Could you check a few things on this drawing? It's one solid part, dimensions in mm from its lowest x, y, z. Give positions to 0.01 mm unless a question says otherwise; leave off trailing zeros. Loops run counter-clockwise (first coordinate to the right, second up) from the corner with the lowest first, then second, coordinate; pieces in that order, holes last. Notation, with made-up numbers: M -22.5,-2 L -17.5,-2 A10 cw -17.5,4 Z; hole C 25,30.5 d2. An arc over 180 degrees is marked long. Return JSON: item names as keys, results as strings. Group by question number.
1. Please list where this line runs through material, in increasing order: line 1 (Y direction, x = 31, z = 0.6).
2. For pin 1 (10 mm diameter, centred on x = 127.5, y = 36, fed in from -Z); pin 2 (2 mm diameter, centred on x = 68, y = 32.5, fed in from +Z), each with a flat end and sliding along its axis, tell me the tip position at first contact or that it passes through.
3. If we section it at A-A (y = 34.5): State how many separate pieces and enclosed holes the cut face has.
4. If we section it at B-B (x = 131): Write out the boundary of the cut face in (y, z).
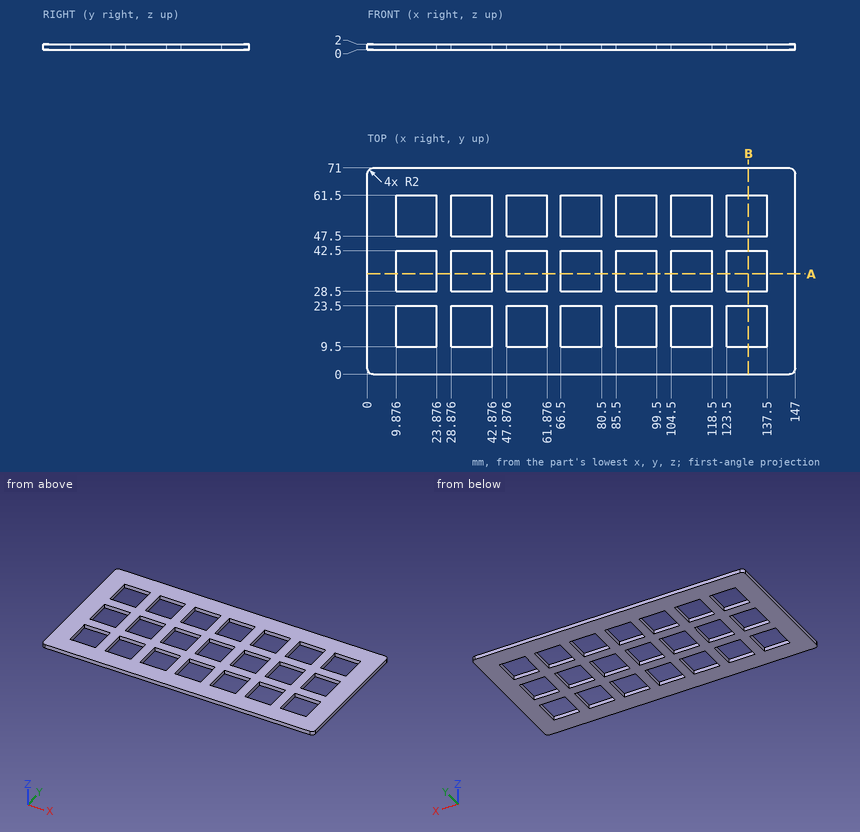
Answer:
{
 "1": {"line 1": "y = 0 to 9.5, 23.5 to 28.5, 42.5 to 47.5, 61.5 to 71"},
 "2": {"pin 1": "stops at z = 0", "pin 2": "passes through"},
 "3": {"separate pieces": "8", "enclosed holes": "0"},
 "4": {"outline": "M 0,0 L 9.5,0 L 9.5,2 L 0,2 Z; M 23.5,0 L 28.5,0 L 28.5,2 L 23.5,2 Z; M 42.5,0 L 47.5,0 L 47.5,2 L 42.5,2 Z; M 61.5,0 L 71,0 L 71,2 L 61.5,2 Z"}
}
